from build123d import *

# Parameters (mm, degrees)
MAIN_PROFILE_SKETCH_R            = 1.1
MAIN_EXTRUSION_DEPTH             = 3
DETAIL_PROFILE_2_SKETCH_R        = 1.1
DETAIL_PROFILE_2_SKETCH_W        = 8
DETAIL_PROFILE_2_SKETCH_H        = 6
DETAIL_EXTRUSION_2_DEPTH         = 0.2
DETAIL_PROFILE_3_SKETCH_R        = 1.6
DETAIL_PROFILE_3_SKETCH_W        = 8
DETAIL_PROFILE_3_SKETCH_H        = 6
DETAIL_EXTRUSION_3_DEPTH         = 2.4
DETAIL_PROFILE_4_SKETCH_R        = 3.2
DETAIL_PROFILE_4_SKETCH_R_2      = 1.6
DETAIL_PROFILE_4_SKETCH_W        = 8
DETAIL_PROFILE_4_SKETCH_H        = 6
DETAIL_EXTRUSION_4_DEPTH         = 1.6
DETAIL_PROFILE_5_SKETCH_W        = 8
DETAIL_PROFILE_5_SKETCH_H        = 6
DETAIL_EXTRUSION_5_DEPTH         = 36.8
DETAIL_PROFILE_6_SKETCH_R        = 1.8
DETAIL_EXTRUSION_6_DEPTH         = 5
CENTRE_BORE_RELIEF_SLOT_SKETCH_W = 9
CENTRE_BORE_RELIEF_SLOT_SKETCH_H = 1.2
CENTRE_BORE_RELIEF_SLOT_DEPTH    = 3.2
ENCODER_CENTRE_OPENING_PROFILE_R = 8
ENCODER_CENTRE_OPENING_DEPTH     = 3.2


with BuildPart() as part:
    # Main Profile Sketch → Main Extrusion (new body)
    with BuildSketch(Plane(origin=(0, -196, 0), x_dir=(-1, 0, 0), z_dir=(0, -1, 0))):
        with BuildLine():
            Line((-14.990817117, 66.244882879), (8.054731733, 66.244882879))
            ThreePointArc((8.054731733, 66.244882879), (12.174217777, 68.810333467), (16.850710954, 70.107296672))
            ThreePointArc((16.850710954, 70.107296672), (19.009182883, 70.944882879), (21.167654813, 70.107296672))
            ThreePointArc((21.167654813, 70.107296672), (36.009182883, 53.244882879), (21.167654813, 36.382469086))
            ThreePointArc((21.167654813, 36.382469086), (20.166826149, 35.761619218), (19.009182883, 35.544882879))
            ThreePointArc((19.009182883, 35.544882879), (17.851539617, 35.761619218), (16.850710954, 36.382469086))
            ThreePointArc((16.850710954, 36.382469086), (7.668676852, 40.580250119), (2.486471241, 49.244882879))
            Line((2.486471241, 49.244882879), (11.009182883, 49.244882879))
            Line((11.009182883, 49.244882879), (11.009182883, 53.244882879))
            Line((11.009182883, 53.244882879), (11.009182883, 57.244882879))
            Line((11.009182883, 57.244882879), (2.486471241, 57.244882879))
            ThreePointArc((2.486471241, 57.244882879), (2.931733644, 58.768977914), (3.517249498, 60.244882879))
            Line((3.517249498, 60.244882879), (-22.990817117, 60.244882879))
            Line((-22.990817117, 60.244882879), (-22.990817117, 68.760672906))
            Line((-22.990817117, 68.760672906), (-14.990817117, 68.760672906))
            Line((-14.990817117, 68.760672906), (-14.990817117, 66.244882879))
        make_face()
        with Locations(Location((19.009182883, 67.744882879, 0), (0, 0, 90))):
            Circle(MAIN_PROFILE_SKETCH_R, mode=Mode.SUBTRACT)
        with Locations(Location((19.009182883, 38.744882879, 0), (0, 0, 90))):
            Circle(MAIN_PROFILE_SKETCH_R, mode=Mode.SUBTRACT)
    extrude(amount=MAIN_EXTRUSION_DEPTH)

    # Detail Profile 2 Sketch → Detail Extrusion 2 (add)
    # profile 1 of 3: a face of its own
    with BuildSketch(Plane(origin=(0, -199, 0), x_dir=(-1, 0, 0), z_dir=(0, -1, 0))):
        with BuildLine():
            Line((16.009182883, 42.994882879), (22.009182883, 42.994882879))
            Line((22.009182883, 42.994882879), (22.009182883, 39.858435751))
            ThreePointArc((22.009182883, 39.858435751), (21.636288628, 36.917777134), (19.009182883, 35.544882879))
            ThreePointArc((19.009182883, 35.544882879), (16.382077138, 36.917777134), (16.009182883, 39.858435751))
            Line((16.009182883, 39.858435751), (16.009182883, 42.994882879))
        make_face()
        with Locations(Location((19.009182883, 38.744882879, 0), (0, 0, 90))):
            Circle(DETAIL_PROFILE_2_SKETCH_R, mode=Mode.SUBTRACT)
    # profile 2 of 3: a face of its own
    with BuildSketch(Plane(origin=(0, -199, 0), x_dir=(-1, 0, 0), z_dir=(0, -1, 0))):
        with Locations((-18.990817117, 65.760672906)):
            Rectangle(DETAIL_PROFILE_2_SKETCH_W, DETAIL_PROFILE_2_SKETCH_H)
    # profile 3 of 3: a face of its own
    with BuildSketch(Plane(origin=(0, -199, 0), x_dir=(-1, 0, 0), z_dir=(0, -1, 0))):
        with BuildLine():
            Line((16.009182883, 66.631330006), (16.009182883, 63.494882879))
            Line((16.009182883, 63.494882879), (22.009182883, 63.494882879))
            Line((22.009182883, 63.494882879), (22.009182883, 66.631330006))
            ThreePointArc((22.009182883, 66.631330006), (19.009182883, 70.944882879), (16.009182883, 66.631330006))
        make_face()
        with Locations(Location((19.009182883, 67.744882879, 0), (0, 0, 90))):
            Circle(DETAIL_PROFILE_2_SKETCH_R, mode=Mode.SUBTRACT)
    extrude(amount=DETAIL_EXTRUSION_2_DEPTH)

    # Detail Profile 3 Sketch → Detail Extrusion 3 (add)
    # profile 1 of 3: a face of its own
    with BuildSketch(Plane(origin=(0, -199.2, 0), x_dir=(-1, 0, 0), z_dir=(0, -1, 0))):
        with BuildLine():
            Line((16.009182883, 42.994882879), (22.009182883, 42.994882879))
            Line((22.009182883, 42.994882879), (22.009182883, 39.858435751))
            ThreePointArc((22.009182883, 39.858435751), (21.636288628, 36.917777134), (19.009182883, 35.544882879))
            ThreePointArc((19.009182883, 35.544882879), (16.382077138, 36.917777134), (16.009182883, 39.858435751))
            Line((16.009182883, 39.858435751), (16.009182883, 42.994882879))
        make_face()
        with Locations(Location((19.009182883, 38.744882879, 0), (0, 0, 90))):
            Circle(DETAIL_PROFILE_3_SKETCH_R, mode=Mode.SUBTRACT)
    # profile 2 of 3: a face of its own
    with BuildSketch(Plane(origin=(0, -199.2, 0), x_dir=(-1, 0, 0), z_dir=(0, -1, 0))):
        with Locations((-18.990817117, 65.760672906)):
            Rectangle(DETAIL_PROFILE_3_SKETCH_W, DETAIL_PROFILE_3_SKETCH_H)
    # profile 3 of 3: a face of its own
    with BuildSketch(Plane(origin=(0, -199.2, 0), x_dir=(-1, 0, 0), z_dir=(0, -1, 0))):
        with BuildLine():
            Line((16.009182883, 66.631330006), (16.009182883, 63.494882879))
            Line((16.009182883, 63.494882879), (22.009182883, 63.494882879))
            Line((22.009182883, 63.494882879), (22.009182883, 66.631330006))
            ThreePointArc((22.009182883, 66.631330006), (19.009182883, 70.944882879), (16.009182883, 66.631330006))
        make_face()
        with Locations(Location((19.009182883, 67.744882879, 0), (0, 0, 90))):
            Circle(DETAIL_PROFILE_3_SKETCH_R, mode=Mode.SUBTRACT)
    extrude(amount=DETAIL_EXTRUSION_3_DEPTH)

    # Detail Profile 4 Sketch → Detail Extrusion 4 (add)
    # profile 1 of 3: a face of its own
    with BuildSketch(Plane(origin=(0, -201.6, 0), x_dir=(-1, 0, 0), z_dir=(0, -1, 0))):
        with Locations(Location((19.009182883, 38.744882879, 0), (0, 0, 227.582921153))):
            Circle(DETAIL_PROFILE_4_SKETCH_R)
        with Locations(Location((19.009182883, 38.744882879, 0), (0, 0, 90))):
            Circle(DETAIL_PROFILE_4_SKETCH_R_2, mode=Mode.SUBTRACT)
    # profile 2 of 3: a face of its own
    with BuildSketch(Plane(origin=(0, -201.6, 0), x_dir=(-1, 0, 0), z_dir=(0, -1, 0))):
        with Locations(Location((19.009182883, 67.744882879, 0), (0, 0, 339.635865194))):
            Circle(DETAIL_PROFILE_4_SKETCH_R)
        with Locations(Location((19.009182883, 67.744882879, 0), (0, 0, 90))):
            Circle(DETAIL_PROFILE_4_SKETCH_R_2, mode=Mode.SUBTRACT)
    # profile 3 of 3: a face of its own
    with BuildSketch(Plane(origin=(0, -201.6, 0), x_dir=(-1, 0, 0), z_dir=(0, -1, 0))):
        with Locations((-18.990817117, 65.760672906)):
            Rectangle(DETAIL_PROFILE_4_SKETCH_W, DETAIL_PROFILE_4_SKETCH_H)
    extrude(amount=DETAIL_EXTRUSION_4_DEPTH)

    # Detail Profile 5 Sketch → Detail Extrusion 5 (add)
    with BuildSketch(Plane(origin=(0, -203.2, 0), x_dir=(-1, 0, 0), z_dir=(0, -1, 0))):
        with Locations((-18.990817117, 65.760672906)):
            Rectangle(DETAIL_PROFILE_5_SKETCH_W, DETAIL_PROFILE_5_SKETCH_H)
    extrude(amount=DETAIL_EXTRUSION_5_DEPTH)

    # Detail Profile 6 Sketch → Detail Extrusion 6 (add)
    with BuildSketch(Plane(origin=(0, -240, 0), x_dir=(-1, 0, 0), z_dir=(0, -1, 0))):
        with BuildLine():
            Line((-22.990817117, 62.760672906), (2.746394057, 62.760672906))
            ThreePointArc((2.746394057, 62.760672906), (6.493392856, 60.960672906), (10.240391655, 62.760672906))
            Line((10.240391655, 62.760672906), (27.777974111, 62.760672906))
            ThreePointArc((27.777974111, 62.760672906), (36.32497291, 65.760672906), (27.777974111, 68.760672906))
            Line((27.777974111, 68.760672906), (10.240391655, 68.760672906))
            ThreePointArc((10.240391655, 68.760672906), (6.493392856, 70.560672906), (2.746394057, 68.760672906))
            Line((2.746394057, 68.760672906), (-22.990817117, 68.760672906))
            Line((-22.990817117, 68.760672906), (-22.990817117, 62.760672906))
        make_face()
        with Locations(Location((31.52497291, 65.760672906, 0), (0, 0, 90))):
            Circle(DETAIL_PROFILE_6_SKETCH_R, mode=Mode.SUBTRACT)
        with Locations(Location((6.493392856, 65.760672906, 0), (0, 0, 90))):
            Circle(DETAIL_PROFILE_6_SKETCH_R, mode=Mode.SUBTRACT)
    extrude(amount=DETAIL_EXTRUSION_6_DEPTH)

    # Centre Bore Relief Slot Sketch → Centre Bore Relief Slot (cut)
    with BuildSketch(Plane(origin=(0, -199.1, 0), x_dir=(1, 0, 0), z_dir=(0, 1, 0))):
        with Locations((-14.509182883, 53.244882879)):
            Rectangle(CENTRE_BORE_RELIEF_SLOT_SKETCH_W, CENTRE_BORE_RELIEF_SLOT_SKETCH_H)
    extrude(amount=CENTRE_BORE_RELIEF_SLOT_DEPTH, mode=Mode.SUBTRACT)

    # Encoder Centre Opening profile → Encoder Centre Opening (cut)
    with BuildSketch(Plane(origin=(0, -199.1, 0), x_dir=(1, 0, 0), z_dir=(0, 1, 0))):
        with Locations((-19.009182883, 53.244882879)):
            Circle(ENCODER_CENTRE_OPENING_PROFILE_R)
    extrude(amount=ENCODER_CENTRE_OPENING_DEPTH, mode=Mode.SUBTRACT)


solid = part.part
Geometry check sheet. Reference: the model listing, model coordinates, mm. A direction names the side the tool comes from. Round coordinates to 2 decimals unless told otherwise and drop trailing zeros. Write each loop counter-clockwise with the first axis right and the second up, starting at its lowest first coordinate (ties: lowest second). Pieces come first, ordered by that corner, then holes. Notation, with made-up numbers: (27, -5.5) -> (39, -5.5) arc R11 ccw to (39, 5.5) -> close; hole circle Ø4 at (68, -22). An arc over 180 degrees is marked (long way). One line per item, written item: value. Start each with the question number.
(1) Cross-section at A-A, the plane x = 1. Record the cut outline in (y, z), and give its area (3 significant figures).
(2) Draft check along X on faces 1 (the flat face through (-11.009, -197, -56)), 2 (the flat face through (-19, -201.6, -64)), 3 (the flat face through (16, -226, -68.761)). Enter one of: +X half, -X half, draft (parallel to the pull), parting line (faces both ways), or undercut.
(3) Cross-section at D-D, the plane x = 18. Record the cut outline in (y, z), and give its area (3 significant figures).
(4) Go/stop test with flat-tipped pins: pin 1 Ø2 at (y, z) = (-200.5, -41) entering from -X; pin 2 Ø0.9 at (x, y) = (-7.5, -198) entering from -Z; pin 3 Ø2.5 at (x, z) = (-18.5, -39) entering from -Y. Record where each tip stops, or that it passes through.
(5) Cross-section at C-C, the plane z = -55. Record the cut outline in (x, y), and give its area (3 significant figures).
(6) Access from +Z, -Z, +X, -X, +Y, -Y to the whole of each face (thin tool, end or side, straight path). Record for faces 4 (the flat face through (-19, -200, -42.995)), 5 (the cylindrical face through (-17.66, -201.172, -39.605)), 6 (the flat face through (-19, -242, -62.761)).
(7) Cross-section at B-B, the plane x = -25.5. Record the cut outline in (y, z), and give its area (3 significant figures).
(8) Scan lines: line 1 (X direction, y = -203, z = -66); line 2 (Y direction, x = -32, z = -58); line 3 (Z direction, x = 15.5, y = -217.5). Record each from-to range of solid material in increasing order. Write a range as [from, to].
Answer:
1. outline: (-245, -68.76) -> (-240, -68.76) -> (-240, -62.76) -> (-245, -62.76) -> close; (-199, -66.24) -> (-196, -66.24) -> (-196, -60.24) -> (-199, -60.24) -> close
1. area: 48.0 mm²
2. face 1: +X half
2. face 2: undercut
2. face 3: draft
3. outline: (-245, -68.76) -> (-196, -68.76) -> (-196, -60.24) -> (-199, -60.24) -> (-199, -62.76) -> (-245, -62.76) -> close
3. area: 302 mm²
4. pin 1: x = -22.01
4. pin 2: z = -66.24
4. pin 3: y = -203.2
5. outline: (-35.92, -199) -> (-26.81, -199) -> (-26.81, -196) -> (-35.92, -196) -> close; (-11.2, -199) -> (-11.01, -199) -> (-11.01, -196) -> (-11.2, -196) -> close
5. area: 27.9 mm²
6. face 4: +X, -X, -Y
6. face 5: -Y
6. face 6: +Z, -Y
7. outline: (-245, -68.76) -> (-240, -68.76) -> (-240, -62.76) -> (-245, -62.76) -> close; (-199, -68.96) -> (-196, -68.96) -> (-196, -57.92) -> (-199, -57.92) -> close; (-199, -48.57) -> (-196, -48.57) -> (-196, -37.53) -> (-199, -37.53) -> close
7. area: 96.2 mm²
8. line 1: [-21.69, -16.33], [14.99, 22.99]
8. line 2: [-199, -196]
8. line 3: [-68.76, -62.76]
